```python
from build123d import *

# Parameters (mm, degrees)
ESQUISSE1_W             = 40
ESQUISSE1_H             = 80
ESQUISSE1_R             = 10
BOSS_EXTRU_1_DEPTH      = 5
ESQUISSE2_R             = 15.5
ENL_V_MAT_EXTRU_1_DEPTH = 1
ESQUISSE3_R             = 1.5
ENL_V_MAT_EXTRU_2_DEPTH = 213.190951739


with BuildPart() as part:
    # Esquisse1 → Boss.-Extru.1 (new body)
    with BuildSketch(Plane.XY):
        Polygon((112.625631329, 137.374368671), (100, 150), (-100, 150), (-112.625631329, 137.374368671), (-98.483495706, 123.232233047), (-123.232233047, 98.483495706), (-137.374368671, 112.625631329), (-150, 100), (-150, -100), (-137.374368671, -112.625631329), (-123.232233047, -98.483495706), (-98.483495706, -123.232233047), (-112.625631329, -137.374368671), (-100, -150), (100, -150), (112.625631329, -137.374368671), (98.483495706, -123.232233047), (123.232233047, -98.483495706), (137.374368671, -112.625631329), (150, -100), (150, 100), (137.374368671, 112.625631329), (123.232233047, 98.483495706), (98.483495706, 123.232233047), align=None)
        with Locations((-90, 0)):
            Rectangle(ESQUISSE1_W, ESQUISSE1_H, mode=Mode.SUBTRACT)
        with Locations((0, -130)):
            Circle(ESQUISSE1_R, mode=Mode.SUBTRACT)
        with Locations((90, 0)):
            Rectangle(ESQUISSE1_W, ESQUISSE1_H, mode=Mode.SUBTRACT)
        with Locations((0, 130)):
            Circle(ESQUISSE1_R, mode=Mode.SUBTRACT)
    extrude(amount=BOSS_EXTRU_1_DEPTH)

    # Esquisse2 → Enlèv. mat.-Extru.1 (cut)
    with BuildSketch(Plane.XY.offset(5)):
        with Locations((0, 130)):
            Circle(ESQUISSE2_R)
        with Locations(Location((0, -130, 0), (0, 0, 180))):
            Circle(ESQUISSE2_R)
    extrude(amount=-ENL_V_MAT_EXTRU_1_DEPTH, mode=Mode.SUBTRACT)

    # Esquisse3 → Enlèv. mat.-Extru.2 (cut, through all)
    with BuildSketch(Plane(origin=(0, 0, 0), x_dir=(-1, 0, 0), z_dir=(0, 0, -1))):
        with Locations((-40.5, 8.042853971)):
            Circle(ESQUISSE3_R)
        with Locations((-40.5, -8.042853971)):
            Circle(ESQUISSE3_R)
        with Locations((-54, 8.042853971)):
            Circle(ESQUISSE3_R)
        with Locations((-54, -8.042853971)):
            Circle(ESQUISSE3_R)
        with Locations((40.5, -8.042853971)):
            Circle(ESQUISSE3_R)
        with Locations((54, -8.042853971)):
            Circle(ESQUISSE3_R)
        with Locations((54, 8.042853971)):
            Circle(ESQUISSE3_R)
        with Locations((40.5, 8.042853971)):
            Circle(ESQUISSE3_R)
    extrude(amount=-ENL_V_MAT_EXTRU_2_DEPTH, mode=Mode.SUBTRACT)


solid = part.part
```
CAD build for the part. Positions are in the model's coordinates, mm. A direction names the side the tool comes from. Give positions to 0.01 mm unless a question says otherwise; leave off trailing zeros. Order: outer loops, then holes, each group sorted by start corner. A loop starts at its lowest first (then second) coordinate and runs counter-clockwise, first axis right, second up. Notation, with made-up numbers: M 38.25,19 L 83.25,19 A22 cw 83.25,46 Z; hole C -35,-25.75 d2. An arc over 180 degrees is marked long. Put each result on its own line as item: value. Start each with the question number.
(1) Saw through at B-B, the plane x = 0. Write the cut outline in (y, z), then the cut area to 3 significant figures.
(2) Which spindle directions (+Z, -Z, +X, -X, +Y, -Y) get a long thin tool onto all of the face, cutting with end or side? Do faces 1 (the flat face through (-105.456, -130.204, 2.465)), 2 (the flat face through (-3, -120, 4)), 3 (the flat face through (105.456, 130.204, 2.465)), 4 (the flat face through (-111.031, -110.685, 2.465)), 5 (the flat face through (-130.204, 105.456, 2.465)). Say none if no direction does.
(3) Saw through at A-A, the plane y = 18.5. Write the cut outline in (x, z).
(4) Drill centre lines: line 1 along Y through (x, z) = (0, 1); line 2 along Y through (x, z) = (54, 2.6); line 3 along X through (y, z) = (26.5, 2.4). Where is each one in solid material? Low to high.
(5) Saw through at C-C, the plane x = 105.5. Write the cut outline in (y, z), then the cut area to 3 significant figures.
(6) Saw through at D-D, the plane y = 130. Write the cut outline in (x, z).
(7) Flat gauge pin, fed straight in: pin 1 Ø4 at (x, y) = (73.5, -21.5) entering from +Z. Where does the tip first touch, or does it go through?
Check result:
1. outline: M -150,0 L -140,0 L -140,4 L -145.5,4 L -145.5,5 L -150,5 Z; M -120,0 L 120,0 L 120,4 L 114.5,4 L 114.5,5 L -114.5,5 L -114.5,4 L -120,4 Z; M 140,0 L 150,0 L 150,5 L 145.5,5 L 145.5,4 L 140,4 Z
1. area: 1,280 mm2
2. face 1: +Z, -Z, -X
2. face 2: +Z
2. face 3: +Z, -Z, +X
2. face 4: +Z, -Z
2. face 5: +Z, -Z, +Y
3. outline: M -150,0 L -110,0 L -110,5 L -150,5 Z; M -70,0 L 70,0 L 70,5 L -70,5 Z; M 110,0 L 150,0 L 150,5 L 110,5 Z
4. line 1: y = -150 to -140, -120 to 120, 140 to 150
4. line 2: y = -150 to -9.54, -6.54 to 6.54, 9.54 to 150
4. line 3: x = -150 to -110, -70 to 70, 110 to 150
5. outline: M -144.5,0 L -130.25,0 L -130.25,5 L -144.5,5 Z; M -116.22,0 L -40,0 L -40,5 L -116.22,5 Z; M 40,0 L 116.22,0 L 116.22,5 L 40,5 Z; M 130.25,0 L 144.5,0 L 144.5,5 L 130.25,5 Z
5. area: 905 mm2
6. outline: M -105.25,0 L -10,0 L -10,4 L -15.5,4 L -15.5,5 L -105.25,5 Z; M 10,0 L 105.25,0 L 105.25,5 L 15.5,5 L 15.5,4 L 10,4 Z
7. pin 1: passes through
